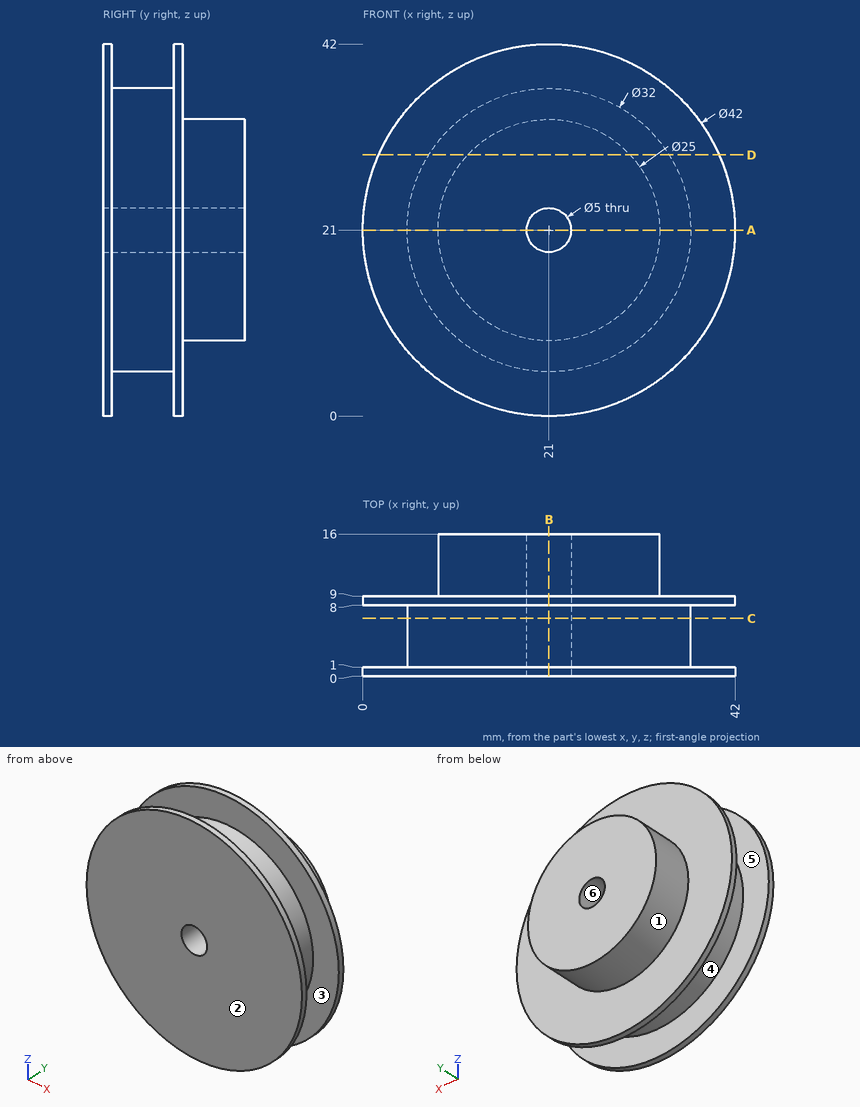
Can you work these out from the drawing? Everything is in mm from the part's minimum corner. A direction names the side the tool comes from. Coordinates: 2 decimals unless noted, no trailing zeros. Loops run counter-clockwise (first coordinate to the right, second up) from the corner with the lowest first, then second, coordinate; pieces in that order, holes last. Notation, with made-up numbers: (29.25, 50.5) -> (68.25, 50.5) arc R36 cw to (68.25, 87.5) -> close; hole circle Ø3 at (47.5, 8). An arc over 180 degrees is marked (long way). Return JSON: item names as keys, results as strings.
1) If we section it at A-A, the plane z = 21: Write out the boundary of the cut face in (x, y), then the cut area to 3 significant figures.
Results below:
{"outline": "(0, 0) -> (18.5, 0) -> (18.5, 16) -> (8.5, 16) -> (8.5, 9) -> (0, 9) -> (0, 8) -> (5, 8) -> (5, 1) -> (0, 1) -> close; (23.5, 0) -> (42, 0) -> (42, 1) -> (37, 1) -> (37, 8) -> (42, 8) -> (42, 9) -> (33.5, 9) -> (33.5, 16) -> (23.5, 16) -> close", "area": "403 mm²"}
2) Thinking about a two-plate mould opening in Z: for the marked faces 4, 5 and 6, which applies, +Z half, -Z half, draft (parallel to the pull), parting line (faces both ways), or undercut?
Results below:
{"face 4": "parting line", "face 5": "draft", "face 6": "undercut"}
3) I need wall thicknesses on line 1 (X direction, y = 12.25, z = 21); line 2 (Z direction, x = 21, y = 7.25); line 3 (Y direction, x = 28.5, z = 37). Which ranges of each line are inside material? Lowest first, please. Write a range as from..to.
Results below:
{"line 1": "8.5..18.5, 23.5..33.5", "line 2": "5..18.5, 23.5..37", "line 3": "0..1, 8..9"}
4) Will these pins go through, and if not, where does the flat tip stop? pin 1 (4 mm diameter, centred on y = 12.5, z = 10, fed in from +X); pin 2 (1 mm diameter, centred on y = 10, z = 16, fed in from -X); pin 3 (1 mm diameter, centred on x = 20, y = 3.5, fed in from +Z).
Results below:
{"pin 1": "x = 29.67", "pin 2": "x = 9.34", "pin 3": "z = 36.99"}
5) If we section it at C-C, the plane y = 6.5: Write out the boundary of the cut face in (x, z), then the cut area to 3 significant figures.
Results below:
{"outline": "circle Ø32 at (21, 21); hole circle Ø5 at (21, 21)", "area": "785 mm²"}
6) If we section it at B-B, the plane x = 21: Write out the boundary of the cut face in (y, z).
Results below:
{"outline": "(0, 0) -> (1, 0) -> (1, 5) -> (8, 5) -> (8, 0) -> (9, 0) -> (9, 8.5) -> (16, 8.5) -> (16, 18.5) -> (0, 18.5) -> close; (0, 23.5) -> (16, 23.5) -> (16, 33.5) -> (9, 33.5) -> (9, 42) -> (8, 42) -> (8, 37) -> (1, 37) -> (1, 42) -> (0, 42) -> close"}
7) If we section it at D-D, the plane z = 29.5: Write out the boundary of the cut face in (x, y).
Results below:
{"outline": "(1.8, 0) -> (40.2, 0) -> (40.2, 1) -> (34.56, 1) -> (34.56, 8) -> (40.2, 8) -> (40.2, 9) -> (30.17, 9) -> (30.17, 16) -> (11.83, 16) -> (11.83, 9) -> (1.8, 9) -> (1.8, 8) -> (7.44, 8) -> (7.44, 1) -> (1.8, 1) -> close"}
8) For the marked faces 1, 2 and 3, which set-ups out of +Z, -Z, +X, -X, +Y, -Y let a thin tool reach every point of the face, with its end or its side?
Results below:
{"face 1": "+Y", "face 2": "+Z, -Z, +X, -X, -Y", "face 3": "none"}
